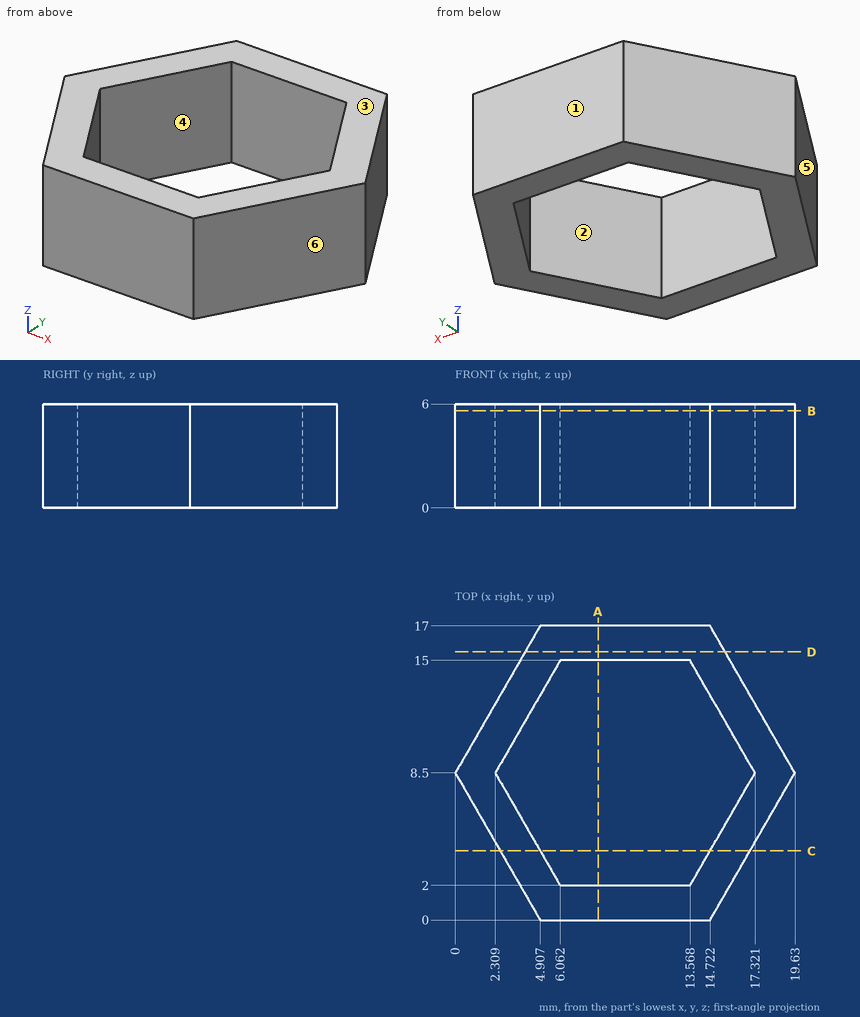
Verification items for this drawing (mm, ordinates from the low corner). A direction names the side the tool comes from. Round coordinates to 2 decimals unless told otherwise and drop trailing zeros. Order: outer loops, then holes, each group sorted by start corner. A loop starts at its lowest first (then second) coordinate and runs counter-clockwise, first axis right, second up. Notation, with made-up numbers: (78.5, 72) -> (113.5, 72) arc R23 cw to (113.5, 94) -> close; hole circle Ø4 at (89.25, 1.25). An arc over 180 degrees is marked (long way). Use one line per item in the form item = value.
1. Cross-section at C-C, the plane y = 4. Enter the section's corners in (x, z), plus the area to 3 significant figures.
Working result:
outline = (2.6, 0) -> (4.91, 0) -> (4.91, 6) -> (2.6, 6) -> close; (14.72, 0) -> (17.03, 0) -> (17.03, 6) -> (14.72, 6) -> close
area = 27.7 mm^2
2. Scan lines: line 1 along Y through (x, z) = (6.5, 2.2); line 2 along Y through (x, z) = (3.25, 3.2) (1 decimal); line 3 along X through (y, z) = (8.75, 0.45) (1 decimal). Record each from-to range of solid material in increasing order. Write a range as from..to.
Working result:
line_1 = 0..2, 15..17
line_2 = 2.9..6.9, 10.1..14.1
line_3 = 0.1..2.5, 17.2..19.5
3. Cross-section at B-B, the plane z = 5.6. Enter the section's corners in (x, y), plus the area to 3 significant figures.
Working result:
outline = (0, 8.5) -> (4.91, 0) -> (14.72, 0) -> (19.63, 8.5) -> (14.72, 17) -> (4.91, 17) -> close; hole (2.31, 8.5) -> (6.06, 2) -> (13.57, 2) -> (17.32, 8.5) -> (13.57, 15) -> (6.06, 15) -> close
area = 104 mm^2
4. Go/stop test with flat-tipped pins: pin 1 (2 mm diameter, centred on y = 10.5, z = 2, fed in from +X); pin 2 (1.5 mm diameter, centred on x = 17.5, y = 14, fed in from +Z). Record where each tip stops, or that it passes through.
Working result:
pin_1 = 19.05
pin_2 = through
5. Mould release check, pull along X, two halves, no side actions. Record for the marked faces 3, 4, 5 and 6: pulls with the +X half, pulls with the -X half, needs draft (parallel to the pull), parting line crosses it, or undercut.
Working result:
face_3 = needs draft
face_4 = undercut
face_5 = pulls with the -X half
face_6 = pulls with the +X half
6. Cross-section at D-D, the plane y = 15.5. Enter the section's corners in (x, z).
Working result:
outline = (4.04, 0) -> (15.59, 0) -> (15.59, 6) -> (4.04, 6) -> close
7. Set-up check for the marked faces 1 and 2: record each of +Z, -Z, +X, -X, +Y, -Y from which the full face is reachable in a straight line by a thin tool's end or side.
Working result:
face_1 = +Z, -Z, +X, -X, +Y
face_2 = +Z, -Z
8. Cross-section at A-A, the plane x = 8.25. Enter the section's corners in (y, z).
Working result:
outline = (0, 0) -> (2, 0) -> (2, 6) -> (0, 6) -> close; (15, 0) -> (17, 0) -> (17, 6) -> (15, 6) -> close
